Read the model definition and answer for the solid it produces. Units are mm, in the model's axes. A direction names the side the tool comes from. Coordinates: 2 decimals unless noted, no trailing zeros. Write each loop counter-clockwise with the first axis right and the second up, starting at its lowest first coordinate (ties: lowest second). Pieces come first, ordered by that corner, then holes. Notation, with made-up numbers: (4, 13) - (39, 13) arc R27 cw to (39, 52) - close; hole circle Ø2 at (-2, 58). An arc over 180 degrees is marked (long way). Return JSON: item names as keys, results as strings.
```python
from build123d import *

# Parameters (mm, degrees)
CROQUIS1_R              = 2.75
CROQUIS1_R_2            = 17.525
SALIENTE_EXTRUIR1_DEPTH = 14.05
CROQUIS3_R              = 20
CROQUIS3_R_2            = 15
SALIENTE_EXTRUIR2_DEPTH = 3


with BuildPart() as part:
    # Croquis1 → Saliente-Extruir1 (new body)
    with BuildSketch(Plane.XY):
        with BuildLine():
            Line((-99.001786664, 30.959159172), (-145.291786664, 30.959159172))
            ThreePointArc((-145.291786664, 30.959159172), (-150.139003649, 28.951376157), (-152.146786664, 24.104159172))
            Line((-152.146786664, 24.104159172), (-152.146786664, -22.185840828))
            ThreePointArc((-152.146786664, -22.185840828), (-150.139003649, -27.033057813), (-145.291786664, -29.040840828))
            Line((-145.291786664, -29.040840828), (-99.001786664, -29.040840828))
            ThreePointArc((-99.001786664, -29.040840828), (-94.154569679, -27.033057813), (-92.146786664, -22.185840828))
            Line((-92.146786664, -22.185840828), (-92.146786664, 24.104159172))
            ThreePointArc((-92.146786664, 24.104159172), (-94.154569679, 28.951376157), (-99.001786664, 30.959159172))
        make_face()
        with Locations((-145.291786664, 24.104159172)):
            Circle(CROQUIS1_R, mode=Mode.SUBTRACT)
        with Locations((-145.291786664, -22.185840828)):
            Circle(CROQUIS1_R, mode=Mode.SUBTRACT)
        with Locations((-99.001786664, -22.185840828)):
            Circle(CROQUIS1_R, mode=Mode.SUBTRACT)
        with Locations((-99.001786664, 24.104159172)):
            Circle(CROQUIS1_R, mode=Mode.SUBTRACT)
        with Locations((-122.146786664, 0.959159172)):
            Circle(CROQUIS1_R_2, mode=Mode.SUBTRACT)
    extrude(amount=SALIENTE_EXTRUIR1_DEPTH)

    # Croquis3 → Saliente-Extruir2 (add)
    with BuildSketch(Plane(origin=(0, 0, 0), x_dir=(-1, 0, 0), z_dir=(0, 0, -1))):
        with Locations((122.146786664, 0.959159172)):
            Circle(CROQUIS3_R)
        with Locations((122.146786664, 0.959159172)):
            Circle(CROQUIS3_R_2, mode=Mode.SUBTRACT)
    extrude(amount=-SALIENTE_EXTRUIR2_DEPTH)


solid = part.part
```
(1) A cutting plane is placed at A-A (y = 13). Determine the outline of the cut face in (x, z).
Answer:
{"outline": "(-152.15, 0) - (-131.09, 0) - (-131.09, 3) - (-134.88, 3) - (-134.88, 14.05) - (-152.15, 14.05) - close; (-113.2, 0) - (-92.15, 0) - (-92.15, 14.05) - (-109.41, 14.05) - (-109.41, 3) - (-113.2, 3) - close"}
(2) Which of the six approach directions +Z, -Z, +X, -X, +Y, -Y give full straight-line access (tool end or side, diameter ignored) to faces 5 (the face through (-135, 9, 3)), 6 (the face through (-92.147, 1, 7))?
Answer:
{"face 5": "+Z", "face 6": "+Z, -Z, +X, +Y, -Y"}
(3) A cutting plane is placed at B-B (x = -100). Determine the outline of the cut face in (y, z).
Answer:
{"outline": "(-29.04, 0) - (-24.75, 0) - (-24.75, 14.05) - (-29.04, 14.05) - close; (-19.62, 0) - (21.54, 0) - (21.54, 14.05) - (-19.62, 14.05) - close; (26.67, 0) - (30.96, 0) - (30.96, 14.05) - (26.67, 14.05) - close"}
(4) A cutting plane is placed at D-D (x = -109). Determine the outline of the cut face in (y, z).
Answer:
{"outline": "(-29.04, 0) - (-6.26, 0) - (-6.26, 3) - (-10.63, 3) - (-10.63, 14.05) - (-29.04, 14.05) - close; (8.18, 0) - (30.96, 0) - (30.96, 14.05) - (12.55, 14.05) - (12.55, 3) - (8.18, 3) - close"}
(5) A flat-ended cylindrical pin translates along its axis: P1, Ø17.5, axis at x = -129.5, y = 1, coming from the +Z side. Find the tip coordinate at first contact, or state that the pin passes through.
Answer:
{"P1": "z = 3"}
(6) Straight lines are drawn through the part: line 1 (X direction, y = -22, z = 10.75); line 2 (X direction, y = 1.5, z = 10.5); line 3 (X direction, y = -21, z = 13.75). For each, find the intervals that lie inside material, in ascending order. Write a range as from..to.
Answer:
{"line 1": "-152.15..-148.04, -142.55..-101.75, -96.26..-92.15", "line 2": "-152.15..-139.66, -104.63..-92.15", "line 3": "-152.15..-147.77, -142.81..-101.48, -96.52..-92.15"}
(7) A cutting plane is placed at C-C (z = 1.25). Determine the outline of the cut face in (x, y) (3 decimals).
Answer:
{"outline": "(-152.147, -22.186) arc R6.855 ccw to (-145.292, -29.041) - (-99.002, -29.041) arc R6.855 ccw to (-92.147, -22.186) - (-92.147, 24.104) arc R6.855 ccw to (-99.002, 30.959) - (-145.292, 30.959) arc R6.855 ccw to (-152.147, 24.104) - close; hole circle Ø5.5 at (-145.292, -22.186); hole circle Ø5.5 at (-145.292, 24.104); hole circle Ø30 at (-122.147, 0.959); hole circle Ø5.5 at (-99.002, -22.186); hole circle Ø5.5 at (-99.002, 24.104)"}
(8) Determine the mould class of faces 1 (the face through (-136, -4.79, 1.48)), 2 (the face through (-139.655, 1.73, 8.448)), 3 (the face through (-94.21, -27.09, 6.93)), 4 (the face through (-94.102, 28.898, 6.927)) for opening direction Y: +Y half, -Y half, draft (parallel to the pull), parting line (faces both ways), or undercut.
Answer:
{"face 1": "undercut", "face 2": "undercut", "face 3": "-Y half", "face 4": "+Y half"}
